Here's how the part is built. I have some questions about the finished solid (model axes, mm). Coordinates: 2 decimals unless noted, no trailing zeros. Write each loop counter-clockwise with the first axis right and the second up, starting at its lowest first coordinate (ties: lowest second). Pieces come first, ordered by that corner, then holes.
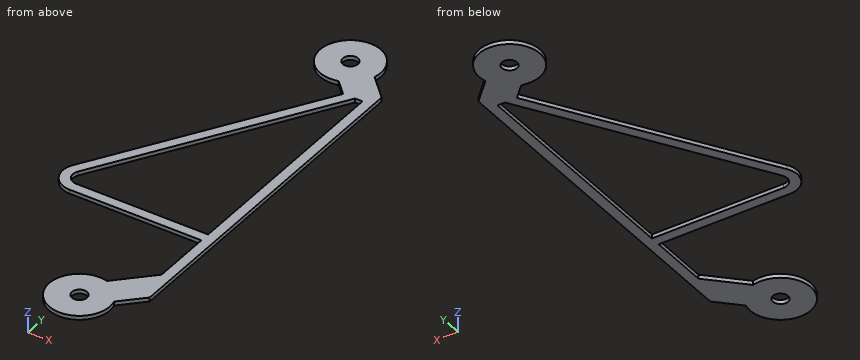
```python
from build123d import *

# Parameters (mm, degrees)
SKETCH1_R           = 0.375
BOSS_EXTRUDE1_DEPTH = 0.1


with BuildPart() as part:
    # Sketch1 → Boss-Extrude1 (new body, symmetric)
    with BuildSketch(Plane.XY):
        with BuildLine():
            Line((1.04409719, 7.895242639), (-5.351162932, -2.475098425))
            ThreePointArc((-5.351162932, -2.475098425), (-5.37318428, -3.487390206), (-4.5, -4))
            Line((-4.5, -4), (2, -4))
            Line((2, -4), (2, -6.939339828))
            Line((2, -6.939339828), (0.388228568, -8.551111261))
            ThreePointArc((0.388228568, -8.551111261), (-1.060660172, -11.060660172), (1.448888739, -9.611771432))
            Line((1.448888739, -9.611771432), (2.5, -8.560660172))
            Line((2.5, -8.560660172), (2.5, 8.560660172))
            Line((2.5, 8.560660172), (1.448888739, 9.611771432))
            ThreePointArc((1.448888739, 9.611771432), (-1.060660172, 11.060660172), (0.388228568, 8.551111261))
            Line((0.388228568, 8.551111261), (1.04409719, 7.895242639))
        make_face()
        with Locations((0, 10)):
            Circle(SKETCH1_R, mode=Mode.SUBTRACT)
        with Locations((0, -10)):
            Circle(SKETCH1_R, mode=Mode.SUBTRACT)
        with BuildLine():
            Line((1.631528786, 7.895242639), (-4.925581466, -2.737549213))
            ThreePointArc((-4.925581466, -2.737549213), (-4.93659214, -3.243695103), (-4.5, -3.5))
            Line((-4.5, -3.5), (2, -3.5))
            Line((2, -3.5), (2, 7.895242639))
            Line((2, 7.895242639), (1.631528786, 7.895242639))
        make_face(mode=Mode.SUBTRACT)
    extrude(amount=BOSS_EXTRUDE1_DEPTH, both=True)


solid = part.part
```
1) Imagine slicing it at A-A on y = -10. Please give me the cut outline in (x, z) (3 decimals), then the cut area to 3 significant figures.
Values follow:
outline: (-1.5, -0.1) - (-0.375, -0.1) - (-0.375, 0.1) - (-1.5, 0.1) - close; (0.375, -0.1) - (1.5, -0.1) - (1.5, 0.1) - (0.375, 0.1) - close
area: 0.450 mm2
2) Imagine slicing it at C-C on x = -2.75. Please give me the cut outline in (y, z), then the cut area to 3 significant figures.
Values follow:
outline: (-4, -0.1) - (-3.5, -0.1) - (-3.5, 0.1) - (-4, 0.1) - close; (0.79, -0.1) - (1.74, -0.1) - (1.74, 0.1) - (0.79, 0.1) - close
area: 0.291 mm2
3) Imagine slicing it at B-B on z = 0. Please give me the cut outline in (x, y) (3 decimals), then the cut area to 3 significant figures.
Values follow:
outline: (-5.351, -2.475) arc R1 ccw to (-4.5, -4) - (2, -4) - (2, -6.939) - (0.388, -8.551) arc R1.5 ccw (long way) to (1.449, -9.612) - (2.5, -8.561) - (2.5, 8.561) - (1.449, 9.612) arc R1.5 ccw (long way) to (0.388, 8.551) - (1.044, 7.895) - close; hole (-4.926, -2.738) arc R0.5 ccw to (-4.5, -3.5) - (2, -3.5) - (2, 7.895) - (1.632, 7.895) - close; hole circle Ø0.75 at (0, -10); hole circle Ø0.75 at (0, 10)
area: 36.0 mm2
4) I need wall thicknesses on probe 1 along X at (y, z) = (-3, 0); probe 2 along Y at (x, z) = (0, 0.05) (3 decimals); probe 3 along Y at (x, z) = (-0.5, 0.05). Which ranges of each line are inside material? Lowest first, please.
Values follow:
probe 1: x = -5.5 to -5, 2 to 2.5
probe 2: y = -11.5 to -10.375, -9.625 to -8.5, -4 to -3.5, 5.25 to 6.202, 8.5 to 9.625, 10.375 to 11.5
probe 3: y = -11.41 to -8.59, -4 to -3.5, 4.44 to 5.39, 8.59 to 11.41
5) Imagine slicing it at D-D on x = 0. Please give me the cut outline in (y, z) (3 decimals), then the cut area to 3 significant figures.
Values follow:
outline: (-11.5, -0.1) - (-10.375, -0.1) - (-10.375, 0.1) - (-11.5, 0.1) - close; (-9.625, -0.1) - (-8.5, -0.1) - (-8.5, 0.1) - (-9.625, 0.1) - close; (-4, -0.1) - (-3.5, -0.1) - (-3.5, 0.1) - (-4, 0.1) - close; (5.25, -0.1) - (6.202, -0.1) - (6.202, 0.1) - (5.25, 0.1) - close; (8.5, -0.1) - (9.625, -0.1) - (9.625, 0.1) - (8.5, 0.1) - close; (10.375, -0.1) - (11.5, -0.1) - (11.5, 0.1) - (10.375, 0.1) - close
area: 1.19 mm2
